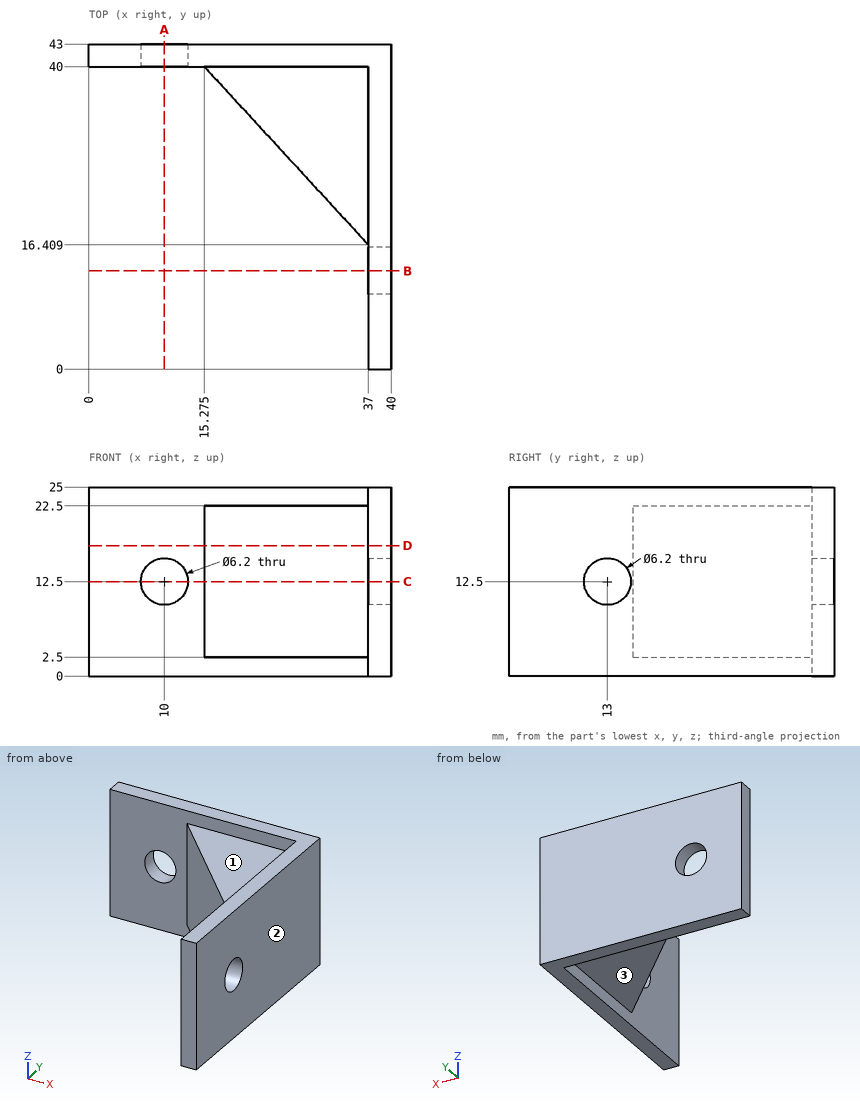
Source: three-view drawing plus pictorial views. Frame: mm from the lowest corner of the part. A direction names the side the tool comes from. Round coordinates to 2 decimals unless told otherwise and drop trailing zeros. Write each loop counter-clockwise with the first axis right and the second up, starting at its lowest first coordinate (ties: lowest second). Pieces come first, ordered by that corner, then holes. Notation, with made-up numbers: M -8,-27.75 L 24,-27.75 A16 cw 24,-2.75 Z; hole C 34,36 d1. An arc over 180 degrees is marked long. Use CSV: the item, a comma, the result in double quotes. Start each with the question number.
Q1. Cut plane B-B on y = 13. Output: boundary loops of the cut face in (x, z), plus the area to 3 significant figures.
Q2. Cut plane D-D on z = 17.25. Output: boundary loops of the cut face in (x, y) (1 decimal), plus the area to 3 significant figures.
Q3. Line query: line 1 (X direction, y = 40.95, z = 12.5); line 2 (X direction, y = 8, z = 1.5); line 3 (Y direction, x = 4.5, z = 9.75). Output: solid intervals per line, ascending. Write a range as from..to.
Q4. Cut plane C-C on z = 12.5. Count the separate pieces of the cut face and the enclosed holes in it, plus the area to 3 significant figures.
Q5. Access query for the marked faces 1, 2 and 3. Directions: +Z, -Z, +X, -X, +Y, -Y. A direction counts if a zero-diameter tool reaches every point of the face in a straight line with its end or side. Return the directions, or none.
Q6. First-contact query: P1, Ø7.5, axis at x = 11, z = 13.5, coming from the -Y side; P2, Ø24, axis at x = 25.5, y = 31.5, coming from the -Z side; P3, Ø4, axis at x = 16, y = 37.5, coming from the +Z side; P4, Ø7.5, axis at y = 25, z = 7, coming from the -X side (1 decimal). Flat tips, straight axial feed; report the tip coordinate or a pass-through.
Q7. Cut plane A-A on x = 10. Output: boundary loops of the cut face in (y, z).
Results found:
1,outline,"M 37,0 L 40,0 L 40,9.4 L 37,9.4 Z; M 37,15.6 L 40,15.6 L 40,25 L 37,25 Z"
1,area,"56.4 mm^2"
2,outline,"M 0,40 L 15.3,40 L 37,16.4 L 37,0 L 40,0 L 40,43 L 0,43 Z"
2,area,"496 mm^2"
3,line 1,"0..6.9, 13.1..40"
3,line 2,"37..40"
3,line 3,"40..43"
4,separate pieces,"3"
4,enclosed holes,"0"
4,area,"459 mm^2"
5,face 1,"+Z, -X, -Y"
5,face 2,"+Z, -Z, +X, +Y, -Y"
5,face 3,"-Z, -X, -Y"
6,P1,"y = 40"
6,P2,"z = 0"
6,P3,"z = 22.5"
6,P4,"x = 25.6"
7,outline,"M 40,0 L 43,0 L 43,9.4 L 40,9.4 Z; M 40,15.6 L 43,15.6 L 43,25 L 40,25 Z"
